The listing builds one solid part. Answer for the finished solid, in the listing's coordinates (mm). A direction names the side the tool comes from. Give positions to 0.01 mm unless a question says otherwise; leave off trailing zeros. Write each loop counter-clockwise with the first axis right and the second up, starting at its lowest first coordinate (ties: lowest second). Pieces come first, ordered by that corner, then holes.
```python
from build123d import *

# Parameters (mm, degrees)
PAD016_DEPTH    = 8
SKETCH023_R     = 2.5
POCKET005_DEPTH = 2
SKETCH024_R     = 2.7
POCKET006_DEPTH = 32.401
POCKET007_DEPTH = 20


with BuildPart() as part:
    # Sketch022 → Pad016 (new body)
    with BuildSketch(Plane.XZ):
        Polygon((-16, 4), (-10, 4), (-10, 5.6), (-1.5, 5.6), (-1.5, 15.6), (1.5, 15.6), (1.5, 5.6), (10, 5.6), (10, 4), (16, 4), (16, 12), (12.975, 15.025), (12.975, 26.950205), (15.975, 30), (15.975, 38), (-15.975, 38), (-15.975, 30), (-12.975, 26.950205), (-12.975, 15.025), (-16, 12), align=None)
    extrude(amount=PAD016_DEPTH)

    # Sketch023 (on Face7 of Pad016) → Pocket005 (cut)
    with BuildSketch(Plane(origin=(0, 0, 5.6), x_dir=(1, 0, 0), z_dir=(0, 0, -1))):
        with Locations((-5, 4)):
            Circle(SKETCH023_R)
        with Locations((5, 4)):
            Circle(SKETCH023_R)
    extrude(amount=-POCKET005_DEPTH, mode=Mode.SUBTRACT)

    # Sketch024 (on Face11 of Pocket005) → Pocket006 (cut, through all)
    with BuildSketch(Plane(origin=(0, 0, 5.6), x_dir=(1, 0, 0), z_dir=(0, 0, -1))):
        with Locations((-5, 4)):
            Circle(SKETCH024_R)
        with Locations((5, 4)):
            Circle(SKETCH024_R)
    extrude(amount=-POCKET006_DEPTH, mode=Mode.SUBTRACT)

    # Sketch025 (on Face19 of Pocket006) → Pocket007 (cut)
    with BuildSketch(Plane(origin=(0, 0, 38), x_dir=(-1, 0, 0), z_dir=(0, 0, 1))):
        with BuildLine():
            ThreePointArc((-6.5, 6.7), (-9.2, 4), (-6.5, 1.3))
            Line((-6.5, 1.3), (-3.5, 1.3))
            ThreePointArc((-3.5, 1.3), (-0.8, 4), (-3.5, 6.7))
            Line((-3.5, 6.7), (-6.5, 6.7))
        make_face()
        with BuildLine():
            ThreePointArc((3.5, 6.7), (0.8, 4), (3.5, 1.3))
            Line((3.5, 1.3), (6.5, 1.3))
            ThreePointArc((6.5, 1.3), (9.2, 4), (6.5, 6.7))
            Line((6.5, 6.7), (3.5, 6.7))
        make_face()
    extrude(amount=-POCKET007_DEPTH, mode=Mode.SUBTRACT)


with BuildPart() as part_1:
    # Body010 placement: moved
    add(part.part.moved(Location((0, -787, 0))))


solid = part_1.part
```
Item 1: A cutting plane is placed at A-A, the plane z = 30.5. Give the vertices of the cut face in (x, y) (3 decimals).
Conclusion:
outline: (-15.975, -795) - (15.975, -795) - (15.975, -787) - (-15.975, -787) - close; hole (-6.5, -793.7) - (-3.5, -793.7) arc R2.7 ccw to (-3.5, -788.3) - (-6.5, -788.3) arc R2.7 ccw to start; hole (3.5, -793.7) - (6.5, -793.7) arc R2.7 ccw to (6.5, -788.3) - (3.5, -788.3) arc R2.7 ccw to start
Item 2: Determine the mould class of faces 5 (the face through (0, -787, 21)), 6 (the face through (-9.2, -790.9, 28.1)), 7 (the face through (-5, -788.3, 28)), 8 (the face through (-13, -791, 4)) for opening direction Y: pulls with the +Y half, pulls with the -Y half, needs draft (parallel to the pull), parting line crosses it, or undercut.
Conclusion:
face 5: pulls with the +Y half
face 6: undercut
face 7: undercut
face 8: needs draft
Item 3: Which of the six approach directions +Z, -Z, +X, -X, +Y, -Y give full straight-line access (tool end or side, diameter ignored) to faces 1 (the face through (5, -793.7, 28)), 2 (the face through (12.975, -791, 21)), 3 (the face through (-10, -791, 5)), 4 (the face through (13, -791, 4))?
Conclusion:
face 1: +Z
face 2: +X, +Y, -Y
face 3: -Z, +Y, -Y
face 4: -Z, +X, -X, +Y, -Y
Item 4: Each of these flat-tipped pins is pushed along its axis until it touches: P1, Ø2.5, axis at y = -789.5, z = 22, coming from the +X side (3 decimals); P2, Ø0.9, axis at x = -0.5, y = -789.5, coming from the -Z side; P3, Ø2, axis at x = -8, y = -790.5, coming from the +Z side; P4, Ø4.5, axis at x = -5, y = -791, coming from the -Z side. Where does it stop, or does it pass through?
Conclusion:
P1: stops at x = 12.975
P2: stops at z = 15.6
P3: stops at z = 18
P4: passes through
Item 5: A cutting plane is placed at D-D, the plane z = 21.5. Give the vertices of the cut face in (x, y) (3 decimals).
Conclusion:
outline: (-12.975, -795) - (12.975, -795) - (12.975, -787) - (-12.975, -787) - close; hole (-6.5, -793.7) - (-3.5, -793.7) arc R2.7 ccw to (-3.5, -788.3) - (-6.5, -788.3) arc R2.7 ccw to start; hole (3.5, -793.7) - (6.5, -793.7) arc R2.7 ccw to (6.5, -788.3) - (3.5, -788.3) arc R2.7 ccw to start
Item 6: A cutting plane is placed at C-C, the plane y = -791. Count the separate pieces of the cut face and the enclosed holes in it, plus the area to 3 significant figures.
Conclusion:
separate pieces: 3
enclosed holes: 0
area: 465 mm2
Item 7: Consider probe 1 along Y at (x, z) = (-5, 35); probe 2 along X at (y, z) = (-791.5, 30) (3 decimals); probe 3 along X at (y, z) = (-790, 22) (3 decimals). Determine where each line is inside the solid, lowest interval first.
Conclusion:
probe 1: y = -795 to -793.7, -788.3 to -787
probe 2: x = -15.975 to -9.153, -0.847 to 0.847, 9.153 to 15.975
probe 3: x = -12.975 to -9.008, -0.992 to 0.992, 9.008 to 12.975
Item 8: A cutting plane is placed at B-B, the plane x = -4.5. Give the vertices of the cut face in (y, z), plus the area to 3 significant figures.
Conclusion:
outline: (-795, 5.6) - (-793.65, 5.6) - (-793.65, 18) - (-793.7, 18) - (-793.7, 38) - (-795, 38) - close; (-788.35, 5.6) - (-787, 5.6) - (-787, 38) - (-788.3, 38) - (-788.3, 18) - (-788.35, 18) - close
area: 85.4 mm2
